Geometry: final body of the model. Coordinates: model frame, mm. Face numbers are marked on the shaded views. Give positions to 0.01 mm unless a question says otherwise; leave off trailing zeros. Write each loop counter-clockwise with the first axis right and the second up, starting at its lowest first coordinate (ties: lowest second). Pieces come first, ordered by that corner, then holes. Notation, with made-up numbers: M -22,69 L 29,69 A22 cw 29,98 Z; hole C -4.5,3 d11. An arc over 180 degrees is marked long. Use a Markdown table: item, result. Add a question column.
(1) Cut plane D-D (z = 6). Output: boundary loops of the cut face in (x, y).
(2) Draft query along X for the marked faces 1, 2, 3 and 4. Return one class per face: released by +X, released by -X, zero draft, split by the parting line, or undercut.
(3) Cut plane A-A (z = 20.5). Output: boundary loops of the cut face in (x, y).
(4) Cut plane B-B (x = 60). Output: boundary loops of the cut face in (y, z), plus the area to 3 significant figures.
(5) Pin query (flat end, axial travel): pin 1 Ø15 at (x, z) = (52, 34.5) entering from -Y; pin 2 Ø4 at (y, z) = (12.5, 57) entering from +X; pin 3 Ø5 at (y, z) = (19, 46.5) entering from +X. Return the tip coordinate at first contact, or that it passes through.
(6) Material intervals for L1, parallel to Z at x = 46, y = 15.5; L2, parallel to Y at x = 50, z = 52, sorted ascending.
(7) Cut plane C-C (y = 10.25). Output: boundary loops of the cut face in (x, z).
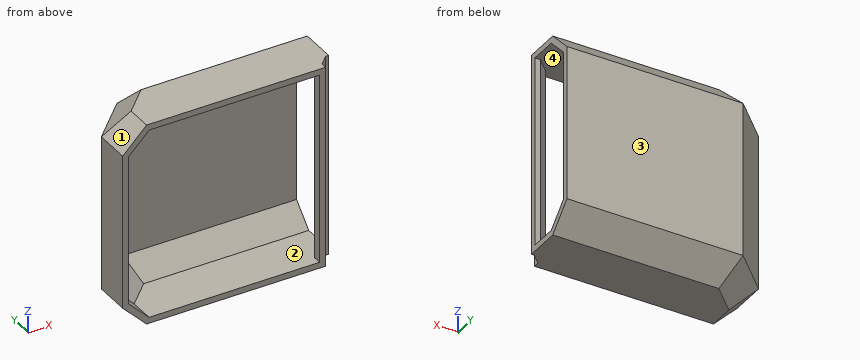
Autodesk Inventor part; units mm, degrees
ref_plane "YZ Plane" through (0, 0, 0) normal (1, 0, 0) x (0, 1, 0)
ref_plane "XZ Plane" through (0, 0, 0) normal (0, 1, 0) x (-1, 0, 0)
ref_plane "XY Plane" through (0, 0, 0) normal (0, 0, 1) x (1, 0, 0)
sketch "Sketch1" plane through (0, 0, 0) normal (0, 0, 1) x (1, 0, 0)
  line L0 (0, 0) -> (0, 12)
  line L1 (0, 12) -> (13, 25)
  line L2 (13, 25) -> (72, 25)
  line L3 (68, 0) -> (68, 2)
  line L4 (68, 2) -> (71, 5)
  line L5 (71, 5) -> (72, 5)
  line L6 (72, 5) -> (72, 25)
  line L7 (68, 0) -> (0, 0)
  point P0 (34, 0)
  dimension "d1" = 45
  dimension "d2" = 25
  dimension "d3" = 68
  dimension "d4" = 5
  dimension "d5" = 2
  dimension "d6" = 12
  dimension "d7" = 38
extrude "Extrusion1" add sketch "Sketch1" along normal blind 68
chamfer "Chamfer1" distance 8 angle 45 6 edges at (0, 6, 68) (6.5, 18.5, 68) (42.5, 25, 68) (0, 6, 0) (6.5, 18.5, 0) (42.5, 25, 0)
shell "Shell1" thickness 2 removed faces 2 at (48, 0, 45.3333) at (72, 11.6667, 25.3333)
properties part number "power_supply_fan_chamber" material "ABS Plastic"
Answer list:
| question | item | result |
|---|---|---|
| 1 | outline | M 2,0 L 4.83,0 L 4.83,10 L 15,20.17 L 72,20.17 L 72,23 L 13.83,23 L 2,11.17 Z; M 66,0 L 68,0 L 68,2 L 71,5 L 72,5 L 72,7 L 70.17,7 L 66,2.83 Z |
| 2 | face 1 | released by -X |
| 2 | face 2 | undercut |
| 2 | face 3 | zero draft |
| 2 | face 4 | undercut |
| 3 | outline | M 0,0 L 2,0 L 2,11.17 L 13.83,23 L 72,23 L 72,25 L 13,25 L 0,12 Z; M 66,0 L 68,0 L 68,2 L 71,5 L 72,5 L 72,7 L 70.17,7 L 66,2.83 Z |
| 4 | outline | M 0,0 L 17,0 L 25,8 L 25,60 L 17,68 L 0,68 L 0,66 L 16.17,66 L 23,59.17 L 23,8.83 L 16.17,2 L 0,2 Z |
| 4 | area | 211 mm² |
| 5 | pin 1 | y = 23 |
| 5 | pin 2 | x = 5.33 |
| 5 | pin 3 | x = 12.33 |
| 6 | L1 | 0 to 2, 66 to 68 |
| 6 | L2 | 23 to 25 |
| 7 | outline | M 0,8 L 4.22,3.78 L 9.56,0 L 72,0 L 72,2 L 10.74,2 L 4.22,6.6 L 2,8.83 L 2,59.17 L 4.22,61.4 L 10.74,66 L 72,66 L 72,68 L 9.56,68 L 4.22,64.22 L 0,60 Z |
